Autodesk Inventor part; units mm, degrees
ref_plane "YZ Plane" through (0, 0, 0) normal (1, 0, 0) x (0, 1, 0)
ref_plane "XZ Plane" through (0, 0, 0) normal (0, 1, 0) x (-1, 0, 0)
ref_plane "XY Plane" through (0, 0, 0) normal (0, 0, 1) x (1, 0, 0)
sketch "Sketch1" plane through (0, 0, 0) normal (0, 0, 1) x (1, 0, 0)
  circle A0 centre (0, 0) radius 40 construction
  circle A1 centre (0, 0) radius 30 construction
  arc A2 (0.0721, 39.6135) -> (0, 40) centre (0, 39.8) ccw
  arc A3 (0.0721, 39.6135) -> (6.0648, 32.2214) centre (1.8749, 34.9497) ccw
  line L0 (6.0648, 32.2214) -> (6.5929, 33.0323)
  line L1 (1.607, 29.9569) -> (7.607, 29.6351) construction
  arc A4 (0, 40) -> (-8.3922, 32.6216) centre (0, 31.5381) ccw
  arc A5 (-17.1227, 35.7218) -> (-17.3553, 36.0388) centre (-17.2686, 35.8586) ccw
  arc A6 (-17.1227, 35.7218) -> (-8.5161, 31.6619) centre (-13.4749, 32.3021) ccw
  line L2 (-8.5161, 31.6619) -> (-8.3922, 32.6216)
  arc A7 (-17.3553, 36.0388) -> (-21.7151, 25.7498) centre (-13.6839, 28.4149) ccw
  arc A8 (-30.9261, 24.755) -> (-31.2733, 24.9396) centre (-31.1169, 24.8149) ccw
  arc A9 (-30.9261, 24.755) -> (-21.4103, 24.8314) centre (-26.1559, 23.2566) ccw
  line L3 (-21.4103, 24.8314) -> (-21.7151, 25.7498)
  arc A10 (-31.2733, 24.9396) -> (-30.7371, 13.778) centre (-24.6575, 19.6637) ccw
  arc A11 (-38.6042, 8.8851) -> (-38.9971, 8.9008) centre (-38.8021, 8.8563) ccw
  arc A12 (-38.6042, 8.8851) -> (-30.064, 13.0827) centre (-33.6563, 9.6049) ccw
  line L4 (-30.064, 13.0827) -> (-30.7371, 13.778)
  arc A13 (-38.9971, 8.9008) -> (-33.6712, -0.9228) centre (-30.7474, 7.0179) ccw
  arc A14 (-38.6363, -8.7445) -> (-38.9971, -8.9008) centre (-38.8021, -8.8563) ccw
  arc A15 (-38.6363, -8.7445) -> (-32.7631, -1.2571) centre (-34.4907, -5.9492) ccw
  line L5 (-32.7631, -1.2571) -> (-33.6712, -0.9228)
  arc A16 (-38.9971, -8.9008) -> (-29.9363, -15.4408) centre (-30.7474, -7.0179) ccw
  arc A17 (-31.016, -24.6422) -> (-31.2733, -24.9396) centre (-31.1169, -24.8149) ccw
  arc A18 (-31.016, -24.6422) -> (-28.9731, -15.348) centre (-28.4938, -20.325) ccw
  line L6 (-28.9731, -15.348) -> (-29.9363, -15.4408)
  arc A19 (-31.2733, -24.9396) -> (-20.2721, -26.9005) centre (-24.6575, -19.6637) ccw
  arc A20 (-17.2526, -35.6592) -> (-17.3553, -36.0388) centre (-17.2686, -35.8586) ccw
  arc A21 (-17.2526, -35.6592) -> (-19.4446, -26.399) centre (-16.8533, -30.6752) ccw
  line L7 (-19.4446, -26.399) -> (-20.2721, -26.9005)
  arc A22 (-17.3553, -36.0388) -> (-6.5929, -33.0323) centre (-13.6839, -28.4149) ccw
  arc A23 (-0.0721, -39.6135) -> (0, -40) centre (0, -39.8) ccw
  arc A24 (-0.0721, -39.6135) -> (-6.0648, -32.2214) centre (-1.8749, -34.9497) ccw
  line L8 (-6.0648, -32.2214) -> (-6.5929, -33.0323)
  arc A25 (0, -40) -> (8.3922, -32.6216) centre (0, -31.5381) ccw
  arc A26 (17.1227, -35.7218) -> (17.3553, -36.0388) centre (17.2686, -35.8586) ccw
  arc A27 (17.1227, -35.7218) -> (8.5161, -31.6619) centre (13.4749, -32.3021) ccw
  line L9 (8.5161, -31.6619) -> (8.3922, -32.6216)
  arc A28 (17.3553, -36.0388) -> (21.7151, -25.7498) centre (13.6839, -28.4149) ccw
  arc A29 (30.9261, -24.755) -> (31.2733, -24.9396) centre (31.1169, -24.8149) ccw
  arc A30 (30.9261, -24.755) -> (21.4103, -24.8314) centre (26.1559, -23.2566) ccw
  line L10 (21.4103, -24.8314) -> (21.7151, -25.7498)
  arc A31 (31.2733, -24.9396) -> (30.7371, -13.778) centre (24.6575, -19.6637) ccw
  arc A32 (38.6042, -8.8851) -> (38.9971, -8.9008) centre (38.8021, -8.8563) ccw
  arc A33 (38.6042, -8.8851) -> (30.064, -13.0827) centre (33.6563, -9.6049) ccw
  line L11 (30.064, -13.0827) -> (30.7371, -13.778)
  arc A34 (38.9971, -8.9008) -> (33.6712, 0.9228) centre (30.7474, -7.0179) ccw
  arc A35 (38.6363, 8.7445) -> (38.9971, 8.9008) centre (38.8021, 8.8563) ccw
  arc A36 (38.6363, 8.7445) -> (32.7631, 1.2571) centre (34.4907, 5.9492) ccw
  line L12 (32.7631, 1.2571) -> (33.6712, 0.9228)
  arc A37 (38.9971, 8.9008) -> (29.9363, 15.4408) centre (30.7474, 7.0179) ccw
  arc A38 (31.016, 24.6422) -> (31.2733, 24.9396) centre (31.1169, 24.8149) ccw
  arc A39 (31.016, 24.6422) -> (28.9731, 15.348) centre (28.4938, 20.325) ccw
  line L13 (28.9731, 15.348) -> (29.9363, 15.4408)
  arc A40 (31.2733, 24.9396) -> (20.2721, 26.9005) centre (24.6575, 19.6637) ccw
  arc A41 (17.2526, 35.6592) -> (17.3553, 36.0388) centre (17.2686, 35.8586) ccw
  arc A42 (17.2526, 35.6592) -> (19.4446, 26.399) centre (16.8533, 30.6752) ccw
  line L14 (19.4446, 26.399) -> (20.2721, 26.9005)
  arc A43 (17.3553, 36.0388) -> (6.5929, 33.0323) centre (13.6839, 28.4149) ccw
  circle A44 centre (0, 0) radius 3.45
  point P0 (-11.55, 27.6875)
  point P1 (-22.4193, 19.9343)
  point P2 (-28.8483, 8.2328)
  point P3 (-29.5634, -5.0993)
  point P4 (-24.4232, -17.4214)
  point P5 (-14.4457, -26.293)
  point P6 (-1.607, -29.9569)
  point P7 (11.55, -27.6875)
  point P8 (22.4193, -19.9343)
  point P9 (28.8483, -8.2328)
  point P10 (29.5634, 5.0993)
  point P11 (24.4232, 17.4214)
  point P12 (14.4457, 26.293)
  point P13 (-8.3922, 32.6216)
  point P14 (-21.7151, 25.7498)
  point P15 (-30.7371, 13.778)
  point P16 (-33.6712, -0.9228)
  point P17 (-29.9363, -15.4408)
  point P18 (-6.5929, -33.0323)
  point P19 (8.3922, -32.6216)
  point P20 (30.7371, -13.778)
  point P21 (33.6712, 0.9228)
  point P22 (29.9363, 15.4408)
  point P23 (20.2721, 26.9005)
  dimension "d14" = 60
  dimension "d6" = 80
  dimension "d16" = 0.2
  dimension "d22" = 5
  dimension "d23" = 60
  dimension "d28" = 6
  dimension "d31" = 360
  dimension "d33" = 6.9
extrude "Extrusion1" add sketch "Sketch1" along normal mid plane 20
properties part number "Turbine"
For this review, take the finished solid that the model builds, in its own axes (mm). Give positions to 0.01 mm unless a question says otherwise; leave off trailing zeros. Write each loop counter-clockwise with the first axis right and the second up, starting at its lowest first coordinate (ties: lowest second). Pieces come first, ordered by that corner, then holes. Notation, with made-up numbers: M 85.5,-36 L 115.5,-36 A17 cw 115.5,-5 Z; hole C 19.5,29.25 d10. An arc over 180 degrees is marked long. Answer as a JSON object with one key per item and string values. Group by question number.
Item 1: Consider section A-A on y = 0. Write out the cut boundary in (x, z).
Item 2: Consider section B-B on x = -25.5. Write out the cut boundary in (y, z).
Item 3: For probe 1 along Y at (x, z) = (0, -1.25); probe 2 along X at (y, z) = (21.5, -0.5); probe 3 along Y at (x, z) = (-34.5, -5.75), list the stretches that pass through material, from the lowest coordinate up. Write a range as [from, to].
Item 4: Draft analysis for pull direction Y (two halves, no side actions). For faces 1 (the cylindrical face through (-38.145, 2.91, -0.14)), 2 (the cylindrical face through (-11.325, -36.541, -0.14)), 3 (the flat face through (8, 1, -10)), 4 (the cylindrical face through (11.325, 36.541, -0.14)), state which applies: +Y half, -Y half, draft (parallel to the pull), parting line (faces both ways), or undercut.
Item 5: For pin 1 Ø11.5 at (x, y) = (13.47, -32.3) entering from +Z; pin 2 Ø8 at (y, z) = (25, 2.5) entering from -X; pin 3 Ø6 at (y, z) = (20.5, 0) entering from -X; pin 4 Ø12 at (y, z) = (1.5, -5.5) entering from +X, all flat-tipped, find the tip position at first contact; note any pin that passes through.
Check result:
{
 "1": {"outline": "M -35.48,-10 L -3.45,-10 L -3.45,10 L -35.48,10 Z; M 3.45,-10 L 35.48,-10 L 35.48,10 L 3.45,10 Z"},
 "2": {"outline": "M -28.08,-10 L -24.33,-10 L -24.33,10 L -28.08,10 Z; M -16.32,-10 L 18.3,-10 L 18.3,10 L -16.32,10 Z"},
 "3": {"probe 1": "y = [-40, -39.58], [-30.31, -3.45], [3.45, 30.31], [39.58, 40]", "probe 2": "x = [-32.92, -30.84], [-21.47, 23.63]", "probe 3": "y = [-14.6, -10.95], [-0.57, 4.68]"},
 "4": {"face 1": "undercut", "face 2": "-Y half", "face 3": "draft", "face 4": "+Y half"},
 "5": {"pin 1": "stops at z = 10", "pin 2": "stops at x = -33.01", "pin 3": "stops at x = -33.12", "pin 4": "stops at x = 38.83"}
}
